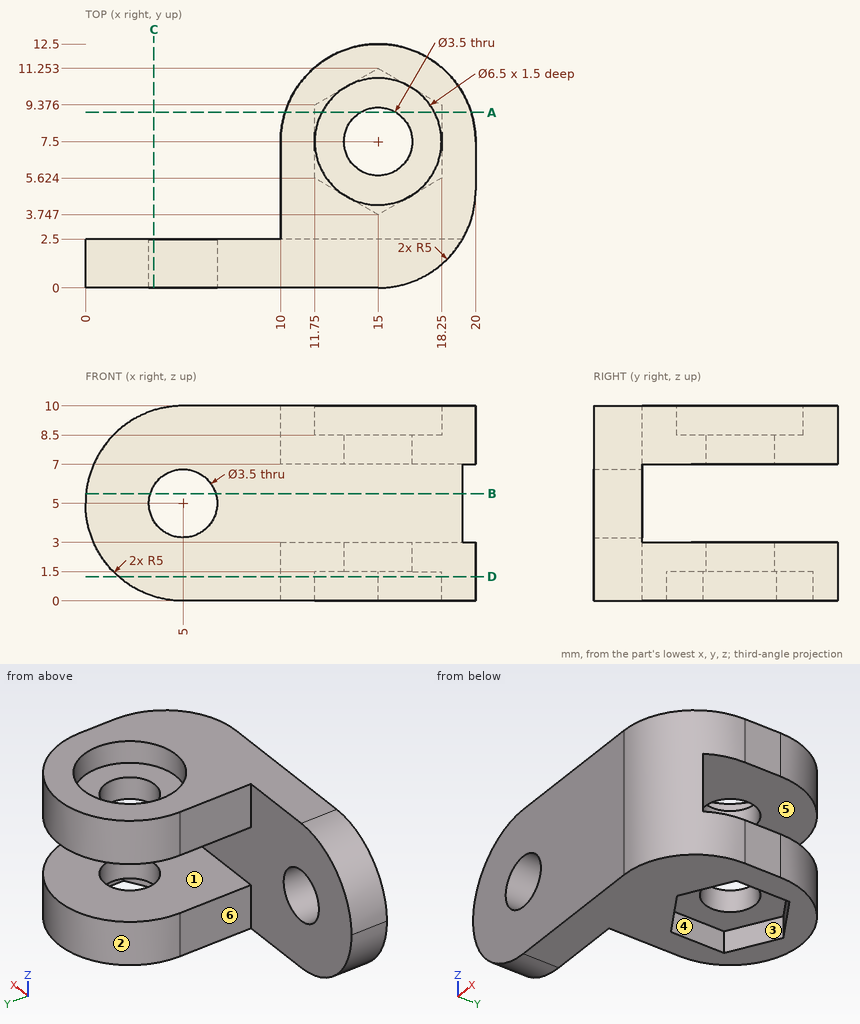
Study the drawing (mm; zero at the part's minimum x, y, z) and answer. A direction names the side the tool comes from. Give positions to 0.01 mm unless a question says otherwise; leave off trailing zeros. Order: outer loops, then holes, each group sorted by start corner. A loop starts at its lowest first (then second) coordinate and runs counter-clockwise, first axis right, second up. Notation, with made-up numbers: (-7.5, -9.5) - (0.5, -9.5) arc R18 ccw to (0.5, 8.5) - close; hole circle Ø4 at (-8.75, 74.25). An arc over 180 degrees is marked (long way). Answer as CSV lines item,"result". Start each with the question number.
Q1. For the marked faces 4, 5 and 6, determine the directions among +Z, -Z, +X, -X, +Y, -Y from which every point of the face is accessible in a straight line to the end or side of a thin tool.
Q2. Given pin 1 Ø6 at (y, z) = (10.5, 7) entering from -X; pin 2 Ø3 at (x, y) = (13.5, 5) entering from +Z; pin 3 Ø4 at (x, y) = (15, 7.5) entering from -Z; pin 4 Ø1 at (x, z) = (7.5, 3) entering from +Y, each flat-ended and moving along its own axis, determine where each tip first touches the part or whether it passes through.
Q3. The part is cut by section C-C (x = 3.5). Write down the section's boundary in (y, z).
Q4. The part is cut by section B-B (z = 5.5). Write down the section's boundary in (x, y) (1 decimal).
Q5. Find the intervals of material crossed by L1, parallel to Z at x = 13, y = 9.5; L2, parallel to X at y = 7.5, z = 2.05; L3, parallel to Z at x = 10.5, y = 6.25, in increasing order. Write a range as [from, to].
Q6. The mould has two halves that part along X. Classify the marked faces 1, 2 and 3: +X half, -X half, draft (parallel to the pull), parting line (faces both ways), or undercut.
Q7. The part is cut by section D-D (z = 1.25). Write down the section's boundary in (x, y).
Q8. The part is cut by section A-A (y = 9). Write down the section's boundary in (x, z).
Check result:
1,face 4,"-Z"
1,face 5,"+X, -X, +Y"
1,face 6,"+Z, -Z, -X, +Y"
2,pin 1,"stops at x = 10"
2,pin 2,"stops at z = 10"
2,pin 3,"stops at z = 1.5"
2,pin 4,"stops at y = 2.5"
3,outline,"(0, 0.23) - (2.5, 0.23) - (2.5, 4.1) - (0, 4.1) - close; (0, 5.9) - (2.5, 5.9) - (2.5, 9.77) - (0, 9.77) - close"
4,outline,"(0, 0) - (3.3, 0) - (3.3, 2.5) - (0, 2.5) - close; (6.7, 0) - (15, 0) arc R5 ccw to (19.3, 2.5) - (6.7, 2.5) - close"
5,L1,"z = [1.5, 3], [7, 8.5]"
5,L2,"x = [10, 13.25], [16.75, 20]"
5,L3,"z = [0, 3], [7, 10]"
6,face 1,"draft"
6,face 2,"parting line"
6,face 3,"undercut"
7,outline,"(1.69, 0) - (15, 0) arc R5 ccw to (20, 5) - (20, 7.5) arc R5 ccw to (10, 7.5) - (10, 2.5) - (1.69, 2.5) - close; hole (11.75, 5.62) - (15, 3.75) - (18.25, 5.62) - (18.25, 9.38) - (15, 11.25) - (11.75, 9.38) - close"
8,outline,"(10.23, 0) - (11.75, 0) - (11.75, 1.5) - (14.1, 1.5) - (14.1, 3) - (10.23, 3) - close; (10.23, 7) - (14.1, 7) - (14.1, 8.5) - (12.12, 8.5) - (12.12, 10) - (10.23, 10) - close; (15.9, 1.5) - (18.25, 1.5) - (18.25, 0) - (19.77, 0) - (19.77, 3) - (15.9, 3) - close; (15.9, 7) - (19.77, 7) - (19.77, 10) - (17.88, 10) - (17.88, 8.5) - (15.9, 8.5) - close"
